The drawing under review shows one solid part. Ordinate dimensions are in mm from its lowest x, y, z. Round coordinates to 2 decimals unless told otherwise and drop trailing zeros. Order: outer loops, then holes, each group sorted by start corner. A loop starts at its lowest first (then second) coordinate and runs counter-clockwise, first axis right, second up. Notation, with made-up numbers: M -31.75,23.5 L 14.25,23.5 A16 cw 14.25,35.5 Z; hole C 87.25,-6.5 d1. An arc over 180 degrees is marked long. Answer as a JSON object with one key per item and string values. Group by question number.
1. Add section B-B on x = 56. State the section outline as (y, z) points (3 decimals), and give its area (3 significant figures).
2. To check wall thickness, follow probe 1 along Y at (x, z) = (69, 4.9) (3 decimals); probe 2 along X at (y, z) = (5, 1.8); probe 3 along X at (y, z) = (28.5, 1.75). State the ranges of each line that lie inside material, in increasing order. Write a range as [from, to].
3. Clearance check with flat-ended pins moving along their axes: P1, Ø10, axis at x = 150, y = 16, coming from the -Z side; P2, Ø1.8, axis at x = 87, z = 3, coming from the +Y side; P3, Ø1.8, axis at y = 82.5, z = 3.5, coming from the -X side. State where each tip first meets the part, or that it passes through.
4. Add section A-A on x = 86.5. State the section outline as (y, z) points (3 decimals).
5. Add section C-C on y = 83.5. State the section outline as (x, z) points.
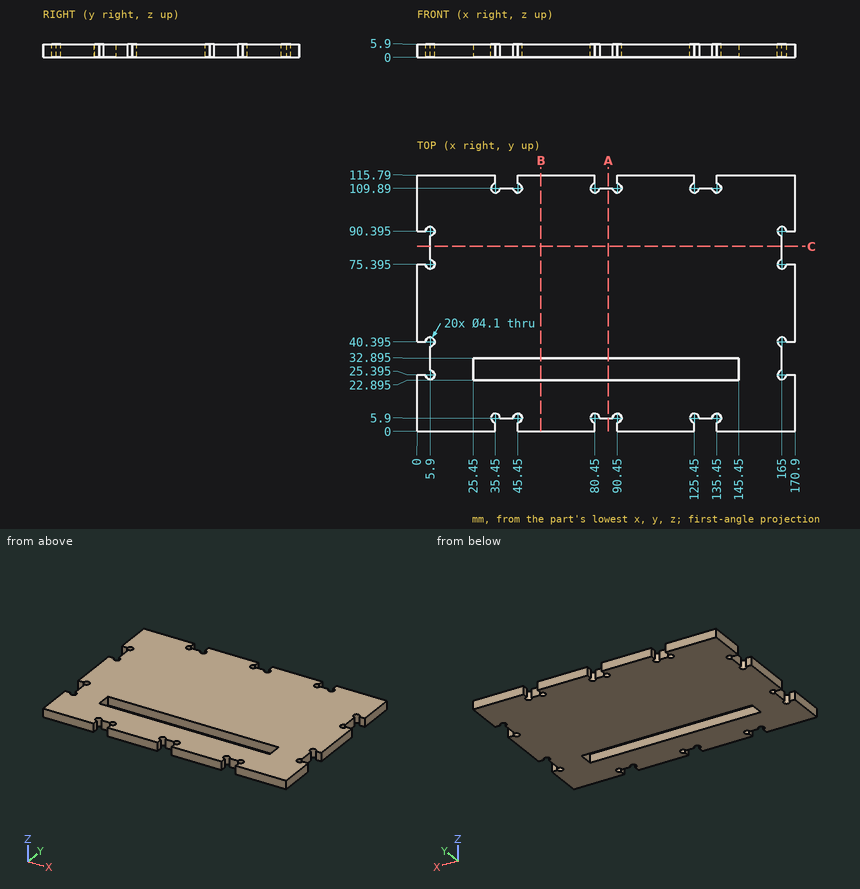
Recorded:
{
 "1": {"outline": "M 0,0 L 22.895,0 L 22.895,5.9 L 0,5.9 Z; M 32.895,0 L 115.79,0 L 115.79,5.9 L 32.895,5.9 Z", "area": "624 mm²"},
 "2": {"probe 1": "y = [0, 22.895], [32.895, 115.79]", "probe 2": "x = [0, 33.61], [47.29, 78.61], [92.29, 123.61], [137.29, 170.9]", "probe 3": "x = [5.9, 25.45], [145.45, 165]"},
 "3": {"P1": "stops at z = 0", "P2": "stops at y = 109.89", "P3": "stops at x = 5.9"},
 "4": {"outline": "M 5.9,0 L 22.895,0 L 22.895,5.9 L 5.9,5.9 Z; M 32.895,0 L 109.89,0 L 109.89,5.9 L 32.895,5.9 Z"},
 "5": {"outline": "M 5.9,0 L 165,0 L 165,5.9 L 5.9,5.9 Z"}
}
